from build123d import *

# Parameters (mm, degrees)
EXTRUDE_1_DEPTH     = 14.5
SKETCH_2_R          = 1
CUT_EXTRUDE_1_DEPTH = 30
CUT_EXTRUDE_START   = -30
SKETCH_3_R          = 1
CUT_EXTRUDE_2_DEPTH = 30
FILLET_1_R          = 2
FILLET_2_R          = 1.5
SKETCH_4_R          = 6.25
SKETCH_4_R_2        = 1.5
CUT_EXTRUDE_3_DEPTH = 30


with BuildPart() as part:
    # ｽｹｯﾁ1 → ﾎﾞｽ - 押し出し1 (new, symmetric)
    with BuildSketch(Plane.XY):
        Polygon((0, 26.298850575), (0, -25.701149425), (22, -25.701149425), (22, -23.701149425), (2, -23.701149425), (2, 24.298850575), (22, 24.298850575), (22, 26.298850575), align=None)
    extrude(amount=EXTRUDE_1_DEPTH, both=True)

    # ｽｹｯﾁ2 → ｶｯﾄ - 押し出し1 (cut)
    with BuildSketch(Plane(origin=(0, 26.298850575, 0), x_dir=(1, 0, 0), z_dir=(0, 1, 0))):
        with BuildLine():
            ThreePointArc((17, 6.25), (10.75, 0), (17, -6.25))
            Line((17, -6.25), (22, -6.25))
            Line((22, -6.25), (22, 6.25))
            Line((22, 6.25), (17, 6.25))
        make_face()
        with Locations(Location((17, 13, 0), (0, 0, 270))):
            Circle(SKETCH_2_R)
        with Locations(Location((17, -13, 0), (0, 0, 270))):
            Circle(SKETCH_2_R)
        with Locations(Location((7, 0, 0), (0, 0, 270))):
            Circle(SKETCH_2_R)
        with Locations(Location((7, 13, 0), (0, 0, 270))):
            Circle(SKETCH_2_R)
        with Locations(Location((7, -13, 0), (0, 0, 270))):
            Circle(SKETCH_2_R)
    extrude(amount=-CUT_EXTRUDE_1_DEPTH, mode=Mode.SUBTRACT)

    # ｽｹｯﾁ3 → ｶｯﾄ - 押し出し2 (cut)
    with BuildSketch(Plane.XZ.offset(25.701149425).offset(CUT_EXTRUDE_START)):
        with BuildLine():
            Line((17, -6.25), (22, -6.25))
            Line((22, -6.25), (22, 6.25))
            Line((22, 6.25), (17, 6.25))
            ThreePointArc((17, 6.25), (10.75, 0), (17, -6.25))
        make_face()
        with Locations(Location((17, -13, 0), (0, 0, 90))):
            Circle(SKETCH_3_R)
        with Locations(Location((17, 13, 0), (0, 0, 90))):
            Circle(SKETCH_3_R)
        with Locations(Location((7, 0, 0), (0, 0, 90))):
            Circle(SKETCH_3_R)
        with Locations(Location((7, -13, 0), (0, 0, 90))):
            Circle(SKETCH_3_R)
        with Locations(Location((7, 13, 0), (0, 0, 90))):
            Circle(SKETCH_3_R)
    extrude(amount=CUT_EXTRUDE_2_DEPTH, mode=Mode.SUBTRACT)

    # ﾌｨﾚｯﾄ1
    fillet_1_edges = [part.edges().sort_by_distance(p)[0] for p in [
        (2, 24.298850575, 0),
        (2, -23.701149425, 0),
        (0, -25.701149425, 0),
        (0, 26.298850575, 0),
    ]]
    fillet(fillet_1_edges, radius=FILLET_1_R)

    # ﾌｨﾚｯﾄ2
    fillet_2_edges = [part.edges().sort_by_distance(p)[0] for p in [
        (22, -24.701149425, -14.5),
        (22, -24.701149425, 14.5),
        (22, 25.298850575, 6.25),
        (22, 25.298850575, -6.25),
        (22, 25.298850575, 14.5),
        (22, 25.298850575, -14.5),
        (22, -24.701149425, 6.25),
        (22, -24.701149425, -6.25),
    ]]
    fillet(fillet_2_edges, radius=FILLET_2_R)

    # ｽｹｯﾁ4 → ｶｯﾄ - 押し出し3 (cut)
    with BuildSketch(Plane.ZY):
        Circle(SKETCH_4_R)
        with Locations((10, -20)):
            Circle(SKETCH_4_R_2)
        with Locations((-10, -20)):
            Circle(SKETCH_4_R_2)
        with Locations((-10, 20)):
            Circle(SKETCH_4_R_2)
        with Locations((10, 20)):
            Circle(SKETCH_4_R_2)
        with Locations((8, -8.5)):
            Circle(SKETCH_4_R_2)
        with Locations((-8, -8.5)):
            Circle(SKETCH_4_R_2)
        with Locations((-8, 8.5)):
            Circle(SKETCH_4_R_2)
        with Locations((8, 8.5)):
            Circle(SKETCH_4_R_2)
    extrude(amount=-CUT_EXTRUDE_3_DEPTH, mode=Mode.SUBTRACT)


solid = part.part
Build history of the part. All positions in model axes, mm. A direction names the side the tool comes from. Round coordinates to 2 decimals unless told otherwise and drop trailing zeros. Write each loop counter-clockwise with the first axis right and the second up, starting at its lowest first coordinate (ties: lowest second). Pieces come first, ordered by that corner, then holes. Notation, with made-up numbers: M -7.5,-31.5 L 16.5,-31.5 A7 ccw 16.5,-18.5 Z; hole C 40.25,88.5 d10. An arc over 180 degrees is marked long. Answer as a JSON object with one key per item and string values. Group by question number.
(1) Cut at B-B (x = 7). Give the number of separate pieces and of enclosed holes in the cut face, and give its area (3 significant figures).
(2) Which spindle directions (+Z, -Z, +X, -X, +Y, -Y) get a long thin tool onto all of the face, cutting with end or side? Do faces 1 (the cylindrical face through (21.57, 25.28, 6.7)), 2 (the flat face through (2, 0, 7)), 3 (the flat face through (22, 25, 10)). Say none if no direction does.
(3) Flat gauge pin, fed straight in: pin 1 (1 mm diameter, centred on y = -18.5, z = 2.5, fed in from +X). Where does the tip first touch, or does it go through?
(4) Drill centre lines: L1, parallel to Y at x = 9.5, z = 10; L2, parallel to Y at x = 0.55, z = 10; L3, parallel to X at y = -24.6, z = -13. Where is each one in solid material? Low to high.
(5) Cut at D-D (z = -0.25). Give the cut face in (x, y) (3 decimals), and give its area (3 significant figures).
(6) Cut at A-A (y = 0). Give the cut face in (x, z), and give its area (3 significant figures).
(7) Cut at C-C (x = 15.25). Give the cut face in (y, z), and give its area (3 significant figures).
(8) Mould opens along Z. For faces 4 (the cylindrical face through (21.55, 25.31, -14.07)), 5 (the flat face through (19, 25, -6.25)), 6 (the flat face through (22, -25, -10)) say: pulls with the +Z half, pulls with the -Z half, needs draft (parallel to the pull), parting line crosses it, or undercut.
Responses:
{
 "1": {"separate pieces": "8", "enclosed holes": "0", "area": "92.0 mm2"},
 "2": {"face 1": "+X, +Y, -Y", "face 2": "+Z, -Z, +X", "face 3": "+Z, -Z, +X, +Y, -Y"},
 "3": {"pin 1": "stops at x = 2"},
 "4": {"L1": "y = -25.7 to -23.7, 24.3 to 26.3", "L2": "y = -25.08 to -21.5, -18.5 to 18.5, 21.5 to 25.68", "L3": "x = 0.21 to 6, 8 to 16, 18 to 22"},
 "5": {"outline": "M 0,-23.701 A2 ccw 2,-25.701 L 6.032,-25.701 L 6.032,-23.701 L 4,-23.701 A2 cw 2,-21.701 L 2,-6.245 L 0,-6.245 Z; M 0,6.245 L 2,6.245 L 2,22.299 A2 cw 4,24.299 L 6.032,24.299 L 6.032,26.299 L 2,26.299 A2 ccw 0,24.299 Z; M 7.968,-25.701 L 10.755,-25.701 L 10.755,-23.701 L 7.968,-23.701 Z; M 7.968,24.299 L 10.755,24.299 L 10.755,26.299 L 7.968,26.299 Z", "area": "106 mm2"},
 "6": {"outline": "M 0,-14.5 L 2,-14.5 L 2,-6.25 L 0,-6.25 Z; M 0,6.25 L 2,6.25 L 2,14.5 L 0,14.5 Z", "area": "33.0 mm2"},
 "7": {"outline": "M -25.7,-14.5 L -23.7,-14.5 L -23.7,-6 L -25.7,-6 Z; M -25.7,6 L -23.7,6 L -23.7,14.5 L -25.7,14.5 Z; M 24.3,-14.5 L 26.3,-14.5 L 26.3,-6 L 24.3,-6 Z; M 24.3,6 L 26.3,6 L 26.3,14.5 L 24.3,14.5 Z", "area": "68.0 mm2"},
 "8": {"face 4": "pulls with the -Z half", "face 5": "undercut", "face 6": "needs draft"}
}
